Part model, mm, in its own coordinate system. A direction names the side the tool comes from. Round coordinates to 2 decimals unless told otherwise and drop trailing zeros. Loops run counter-clockwise (first coordinate to the right, second up) from the corner with the lowest first, then second, coordinate; pieces in that order, holes last. Notation, with made-up numbers: (2, -30.5) -> (51, -30.5) arc R15 ccw to (51, -2.5) -> close; hole circle Ø7 at (16.25, -16.5). An arc over 180 degrees is marked (long way). Answer as CSV lines item,"result".
from build123d import *

# Parameters (mm, degrees)
BOSS_EXTRUDE1_DEPTH = 304.8
CHAMFER1_SIZE       = 304.8
SKETCH3_W           = 304.8
SKETCH3_H           = 1066.8
BOSS_EXTRUDE2_DEPTH = 1529.08
FILLET1_R           = 533.4
BOSS_EXTRUDE3_DEPTH = 152.4


with BuildPart() as part:
    # Sketch1 → Boss-Extrude1 (new body)
    with BuildSketch(Plane(origin=(0, 0, 0), x_dir=(1, 0, 0), z_dir=(0, 1, 0))):
        Polygon((838.2, -228.6), (533.4, -533.4), (-838.2, -533.4), (-838.2, 533.4), (838.2, 533.4), align=None)
    extrude(amount=BOSS_EXTRUDE1_DEPTH)

    # Chamfer1
    chamfer1_edges = [part.edges().sort_by_distance(p)[0] for p in [
        (838.2, 152.4, -533.4),
    ]]
    chamfer(chamfer1_edges, length=CHAMFER1_SIZE)

    # Sketch3 → Boss-Extrude2 (add)
    with BuildSketch(Plane(origin=(0, 304.8, 0), x_dir=(1, 0, 0), z_dir=(0, 1, 0))):
        with Locations((-685.8, 0)):
            Rectangle(SKETCH3_W, SKETCH3_H)
    extrude(amount=BOSS_EXTRUDE2_DEPTH)

    # Fillet1
    fillet1_edges = [part.edges().sort_by_distance(p)[0] for p in [
        (-685.8, 1833.88, -533.4),
        (-685.8, 1833.88, 533.4),
    ]]
    fillet(fillet1_edges, radius=FILLET1_R - 0.0001)  # a hair under: the kernel refuses the full size

    # Sketch4 → Boss-Extrude3 (add, symmetric)
    with BuildSketch(Plane.XY):
        Polygon((-533.4, 1371.6), (838.2, 304.8), (-533.4, 304.8), align=None)
    extrude(amount=BOSS_EXTRUDE3_DEPTH, both=True)


solid = part.part
Q1. Drill centre lines: line 1 along X through (y, z) = (612, 268.5); line 2 along Y through (x, z) = (245.5, -297); line 3 along Z through (x, y) = (15, 586). Where is each one in solid material? Low to high.
Geometry results:
line 1,"-838.2 to -533.4"
line 2,"0 to 304.8"
line 3,"-152.4 to 152.4"
Q2. Drop flat-ended pins along their axis: P1, Ø2, axis at x = 10.5, y = 701, coming from the +Z side; P2, Ø4, axis at y = 1645, z = 338.5, coming from the +X side; P3, Ø1, axis at x = 286, z = -400.5, coming from the +Y side. Give the stop position or say it passes through.
Geometry results:
P1,"z = 152.4"
P2,"x = -533.4"
P3,"y = 304.8"
Q3. Saw through at D-D, the plane y = 773. Write the cut outline in (x, z).
Geometry results:
outline,"(-838.2, -533.4) -> (-533.4, -533.4) -> (-533.4, -152.4) -> (236.23, -152.4) -> (236.23, 152.4) -> (-533.4, 152.4) -> (-533.4, 533.4) -> (-838.2, 533.4) -> close"
Q4. Saw through at A-A, the plane x = -10.5. Write the cut outline in (y, z), then the cut area to 3 significant figures.
Geometry results:
outline,"(0, -533.4) -> (304.8, -533.4) -> (304.8, -152.4) -> (964.9, -152.4) -> (964.9, 152.4) -> (304.8, 152.4) -> (304.8, 533.4) -> (0, 533.4) -> close"
area,"526,000 mm2"
Q5. Saw through at B-B, the plane y = 244. Write the cut outline in (x, z).
Geometry results:
outline,"(-838.2, -533.4) -> (533.4, -533.4) -> (838.2, -228.6) -> (838.2, 228.6) -> (533.4, 533.4) -> (-838.2, 533.4) -> close"
Q6. Two-plate mould, pull along Y, no slides. Class faces 1 (the face through (687.9, 150.3, 378.9)), 2 (the face through (-683.666, 1673.481, -381.295)), 3 (the face through (12, 0, -7)): pulls with the +Y half, pulls with the -Y half, needs draft (parallel to the pull), parting line crosses it, or undercut.
Geometry results:
face 1,"needs draft"
face 2,"pulls with the +Y half"
face 3,"pulls with the -Y half"
Q7. Which spindle directions (+Z, -Z, +X, -X, +Y, -Y) get a long thin tool onto all of the face, cutting with end or side? Do faces 4 (the face through (-143, 609, -152.4)), 5 (the face through (-143, 609, 152.4)), 6 (the face through (-533.4, 1059, -230)). Say none if no direction does.
Geometry results:
face 4,"-Z, +X, +Y"
face 5,"+Z, +X, +Y"
face 6,"+X, +Y"
Q8. Saw through at C-C, the plane z = 379. Write the cut outline in (x, y).
Geometry results:
outline,"(-838.2, 0) -> (687.8, 0) -> (687.8, 304.8) -> (-533.4, 304.8) -> (-533.4, 1675.81) -> (-838.2, 1675.81) -> close"
